from build123d import *
from OCP.BRepFilletAPI import BRepFilletAPI_MakeChamfer
from build123d.topology import SkipClean

# Parameters (mm, degrees)
SKETCH1_R                = 1.6
SKETCH1_W                = 16
SKETCH1_H                = 16
BOSS_EXTRUDE1_DEPTH      = 8
SKETCH2_W                = 16
SKETCH2_H                = 4
CUT_EXTRUDE1_DEPTH       = 40
FILLET1_R                = 4
BOSS_EXTRUDE5_DEPTH      = 12
BOSS_EXTRUDE5_DEPTH_BACK = 1
SKETCH3_W                = 32
SKETCH3_H                = 5
CHAMFER1_SIZE            = 3
CHAMFER2_SIZE            = 8
CHAMFER2_SIZE2           = 10
SKETCH5_W                = 12
SKETCH5_H                = 5
BOSS_EXTRUDE7_DEPTH      = 8
FILLET2_R                = 4
SKETCH6_R                = 1.6
CUT_EXTRUDE2_DEPTH       = 20
SKETCH7_R                = 3.05
CUT_EXTRUDE3_DEPTH       = 9
SKETCH8_R                = 3.05
BOSS_EXTRUDE8_DEPTH      = 5
BOSS_EXTRUDE9_START      = -5
SKETCH9_R                = 1.6
BOSS_EXTRUDE9_DEPTH      = 5
SKETCH10_R               = 5.55
CUT_EXTRUDE4_DEPTH       = 9
BOSS_EXTRUDE11_START     = 6
SKETCH11_R               = 5.55
BOSS_EXTRUDE11_DEPTH     = 6
SKETCH12_R               = 7.71946315
SKETCH12_R_2             = 3.05
BOSS_EXTRUDE12_DEPTH     = 5.5
SKETCH14_R               = 7
CUT_EXTRUDE6_DEPTH       = 1.5
CUT_EXTRUDE8_DEPTH       = 5
BOSS_EXTRUDE13_START     = -6
SKETCH19_R               = 2.06
SKETCH19_R_2             = 7
BOSS_EXTRUDE13_DEPTH     = 6
CUT_EXTRUDE9_DEPTH       = 8
FILLET3_R                = 2
CHAMFER3_SIZE            = 4


# Some blends are built 0.0001 mm under size
with BuildPart() as part:
    # Sketch1 → Boss-Extrude1 (new body)
    with BuildSketch(Plane(origin=(0, 0, 0), x_dir=(1, 0, 0), z_dir=(0, 1, 0))):
        with BuildLine():
            Line((-12, 16), (12, 16))
            ThreePointArc((12, 16), (14.828427125, 14.828427125), (16, 12))
            Line((16, 12), (16, -12))
            ThreePointArc((16, -12), (14.828427125, -14.828427125), (12, -16))
            Line((12, -16), (-12, -16))
            ThreePointArc((-12, -16), (-14.828427125, -14.828427125), (-16, -12))
            Line((-16, -12), (-16, 12))
            ThreePointArc((-16, 12), (-14.828427125, 14.828427125), (-12, 16))
        make_face()
        with Locations(Location((12, 12, 0), (0, 0, 270))):
            Circle(SKETCH1_R, mode=Mode.SUBTRACT)
        with Locations(Location((-12, 12, 0), (0, 0, 90))):
            Circle(SKETCH1_R, mode=Mode.SUBTRACT)
        with Locations(Location((12, -12, 0), (0, 0, 90))):
            Circle(SKETCH1_R, mode=Mode.SUBTRACT)
        with Locations(Location((-12, -12, 0), (0, 0, 270))):
            Circle(SKETCH1_R, mode=Mode.SUBTRACT)
        Rectangle(SKETCH1_W, SKETCH1_H, mode=Mode.SUBTRACT)
    extrude(amount=BOSS_EXTRUDE1_DEPTH)

    # Sketch2 → Cut-Extrude1 (cut)
    with BuildSketch(Plane(origin=(16, 0, 0), x_dir=(0, 0, -1), z_dir=(1, 0, 0))):
        with Locations((0, 2)):
            Rectangle(SKETCH2_W, SKETCH2_H)
    extrude(amount=-CUT_EXTRUDE1_DEPTH, mode=Mode.SUBTRACT)

    # Fillet1
    fillet1_edges = [part.edges().sort_by_distance(p)[0] for p in [
        (-16, 2, -8),
        (16, 2, -8),
        (-16, 2, 8),
        (16, 2, 8),
    ]]
    fillet(fillet1_edges, radius=FILLET1_R - 0.0001)  # a hair under: the kernel refuses the full size

    # Sketch3 → Boss-Extrude5 (add, two sides: drawn at the far end of the back side and taken through both)
    with BuildSketch(Plane(origin=(0, 8, 0), x_dir=(1, 0, 0), z_dir=(0, 1, 0)).offset(-BOSS_EXTRUDE5_DEPTH_BACK)):
        with Locations((0, 5.5)):
            Rectangle(SKETCH3_W, SKETCH3_H)
        with Locations((0, -5.5)):
            Rectangle(SKETCH3_W, SKETCH3_H)
    extrude(amount=BOSS_EXTRUDE5_DEPTH + BOSS_EXTRUDE5_DEPTH_BACK)

    # Chamfer1
    chamfer1_edges = [part.edges().sort_by_distance(p)[0] for p in [
        (8, 7, 5.5),
        (8, 7, -5.5),
        (-8, 7, -5.5),
        (-8, 7, 5.5),
    ]]
    chamfer(chamfer1_edges, length=CHAMFER1_SIZE - 0.0001)  # a hair under: the kernel refuses the full size

    # Chamfer2: one chamfer whose edges measure the first distance from different faces: ONE call of the kernel's chamfer builder (chamfer() names one face for all edges)
    chamfer2_edges_1 = [part.edges().sort_by_distance(p)[0] for p in [
        (-16, 20, -5.5),
        (-16, 20, 5.5),
    ]]
    chamfer2_side_1 = [part.faces().sort_by_distance(p)[0] for p in [
        (-16, 0.312409987, 11.99995),
    ]]
    chamfer2_edges_2 = [part.edges().sort_by_distance(p)[0] for p in [
        (16, 20, -5.5),
        (16, 20, 5.5),
    ]]
    chamfer2_side_2 = [part.faces().sort_by_distance(p)[0] for p in [
        (16, 0.312409987, -11.99995),
    ]]
    chamfer2 = BRepFilletAPI_MakeChamfer(part.part.solid().wrapped)
    for e in chamfer2_edges_1:
        chamfer2.Add(CHAMFER2_SIZE, CHAMFER2_SIZE2, e.wrapped, chamfer2_side_1[0].wrapped)  # the first distance lies on this face
    for e in chamfer2_edges_2:
        chamfer2.Add(CHAMFER2_SIZE, CHAMFER2_SIZE2, e.wrapped, chamfer2_side_2[0].wrapped)  # the first distance lies on this face
    add(Compound.cast(chamfer2.Shape()), mode=Mode.REPLACE)

    # Sketch5 → Boss-Extrude7 (add)
    with BuildSketch(Plane(origin=(0, 20, 0), x_dir=(1, 0, 0), z_dir=(0, 1, 0))):
        with Locations((0, 5.5)):
            Rectangle(SKETCH5_W, SKETCH5_H)
        with Locations((0, -5.5)):
            Rectangle(SKETCH5_W, SKETCH5_H)
    extrude(amount=BOSS_EXTRUDE7_DEPTH)

    # Fillet2
    fillet2_edges = [part.edges().sort_by_distance(p)[0] for p in [
        (-6, 28, -5.5),
        (6, 28, -5.5),
        (-6, 28, 5.5),
        (6, 28, 5.5),
    ]]
    fillet(fillet2_edges, radius=FILLET2_R)

    # Sketch6 → Cut-Extrude2 (cut)
    with BuildSketch(Plane.XY.offset(8)):
        with Locations((0, 24)):
            Circle(SKETCH6_R)
    extrude(amount=-CUT_EXTRUDE2_DEPTH, mode=Mode.SUBTRACT)

    # Sketch7 → Cut-Extrude3 (cut)
    with BuildSketch(Plane.XY.offset(8)):
        with Locations((0, 24)):
            Circle(SKETCH7_R)
    extrude(amount=-CUT_EXTRUDE3_DEPTH, mode=Mode.SUBTRACT)

    # Sketch8 → Boss-Extrude8 (add)
    with BuildSketch(Plane.XY.offset(8)):
        with BuildLine():
            Line((-9, 24), (-9, 15))
            Line((-9, 15), (0, 15))
            Line((0, 15), (9, 15))
            Line((9, 15), (9, 24))
            ThreePointArc((9, 24), (0, 33), (-9, 24))
        make_face()
        with Locations((0, 24)):
            Circle(SKETCH8_R, mode=Mode.SUBTRACT)
    extrude(amount=-BOSS_EXTRUDE8_DEPTH)

    # Sketch9 → Boss-Extrude9 (add)
    with BuildSketch(Plane(origin=(0, 0, -8), x_dir=(-1, 0, 0), z_dir=(0, 0, -1)).offset(BOSS_EXTRUDE9_START)):
        with BuildLine():
            Line((-9, 24), (-9, 11))
            Line((-9, 11), (9, 11))
            Line((9, 11), (9, 24))
            ThreePointArc((9, 24), (0, 33), (-9, 24))
        make_face()
        with Locations(Location((0, 24, 0), (0, 0, 180))):
            Circle(SKETCH9_R, mode=Mode.SUBTRACT)
    extrude(amount=BOSS_EXTRUDE9_DEPTH)

    # Sketch10 → Cut-Extrude4 (cut)
    with BuildSketch(Plane(origin=(0, 0, -8), x_dir=(-1, 0, 0), z_dir=(0, 0, -1))):
        with Locations((0, 24)):
            Circle(SKETCH10_R)
    extrude(amount=-CUT_EXTRUDE4_DEPTH, mode=Mode.SUBTRACT)

    # Sketch11 → Boss-Extrude11 (add)
    with SkipClean():  # the faces are left unmerged after this step: merging them gives an invalid solid
        with BuildSketch(Plane.XY.offset(-3).offset(BOSS_EXTRUDE11_START)):
            with BuildLine():
                Line((-9, 24), (-9, 17.6))
                Line((-9, 17.6), (-16, 12))
                Line((-16, 12), (-16, 8))
                Line((-16, 8), (-8, 8))
                Line((-8, 8), (-8, 4))
                Line((-8, 4), (-5, 7))
                Line((-5, 7), (5, 7))
                Line((5, 7), (8, 4))
                Line((8, 4), (8, 8))
                Line((8, 8), (16, 8))
                Line((16, 8), (16, 12))
                Line((16, 12), (9, 17.6))
                Line((9, 17.6), (9, 24))
                ThreePointArc((9, 24), (0, 33), (-9, 24))
            make_face()
            with Locations(Location((0, 24, 0), (0, 0, 180))):
                Circle(SKETCH11_R, mode=Mode.SUBTRACT)
        extrude(amount=-BOSS_EXTRUDE11_DEPTH)

    # Sketch12 → Boss-Extrude12 (add)
    with BuildSketch(Plane(origin=(0, 0, 3), x_dir=(-1, 0, 0), z_dir=(0, 0, -1))):
        with Locations((0, 24)):
            Circle(SKETCH12_R)
        with Locations(Location((0, 24, 0), (0, 0, 180))):
            Circle(SKETCH12_R_2, mode=Mode.SUBTRACT)
    extrude(amount=BOSS_EXTRUDE12_DEPTH)

    # Sketch14 → Cut-Extrude6 (cut)
    with BuildSketch(Plane(origin=(0, 0, -8), x_dir=(-1, 0, 0), z_dir=(0, 0, -1))):
        with Locations((0, 24)):
            Circle(SKETCH14_R)
    extrude(amount=-CUT_EXTRUDE6_DEPTH, mode=Mode.SUBTRACT)

    # Sketch16 → Cut-Extrude8 (cut)
    with SkipClean():  # the faces are left unmerged after this step: merging them gives an invalid solid
        with BuildSketch(Plane.XY.offset(8)):
            Polygon((-16, 8), (16, 8), (29.507054263, 32.870046285), (-4.901166162, 51.167615183), (-28.978076235, 29.234025221), align=None)
        extrude(amount=-CUT_EXTRUDE8_DEPTH, mode=Mode.SUBTRACT)

    # Sketch19 → Boss-Extrude13 (add)
    with SkipClean():  # the faces are left unmerged after this step: merging them gives an invalid solid
        with BuildSketch(Plane(origin=(0, 0, -8), x_dir=(-1, 0, 0), z_dir=(0, 0, -1)).offset(BOSS_EXTRUDE13_START)):
            with BuildLine():
                Line((16.13, 29), (7.483314774, 29))
                ThreePointArc((7.483314774, 29), (0, 33), (-7.483314774, 29))
                Line((-7.483314774, 29), (-16.13, 29))
                ThreePointArc((-16.13, 29), (-20.352655353, 26.677532777), (-20.652519245, 21.867672708))
                Line((-20.652519245, 21.867672708), (-16, 12))
                Line((-16, 12), (16, 12))
                Line((16, 12), (20.652519245, 21.867672708))
                ThreePointArc((20.652519245, 21.867672708), (20.352655353, 26.677532777), (16.13, 29))
            make_face()
            with Locations((16.13, 24)):
                Circle(SKETCH19_R, mode=Mode.SUBTRACT)
            with Locations(Location((-16.13, 24, 0), (0, 0, 180))):
                Circle(SKETCH19_R, mode=Mode.SUBTRACT)
            with Locations((0, 24)):
                Circle(SKETCH19_R_2, mode=Mode.SUBTRACT)
        extrude(amount=BOSS_EXTRUDE13_DEPTH)

    # Sketch21 → Cut-Extrude9 (cut)
    with SkipClean():  # the faces are left unmerged after this step: merging them gives an invalid solid
        with BuildSketch(Plane(origin=(0, 0, -16), x_dir=(-1, 0, 0), z_dir=(0, 0, -1))):
            with BuildLine():
                Line((8, 8), (0, 8))
                Line((0, 8), (0, 3))
                ThreePointArc((0, 3), (4.716990566, 4.352815094), (8, 8))
            make_face()
            with BuildLine():
                Line((0, 3), (0, 8))
                Line((0, 8), (-8, 8))
                ThreePointArc((-8, 8), (-4.716990566, 4.352815094), (0, 3))
            make_face()
        extrude(amount=-CUT_EXTRUDE9_DEPTH, mode=Mode.SUBTRACT)

    # Fillet3
    # the kernel refuses this fillet: 2 mm, written as the material it takes off along each edge
    with BuildSketch(Plane(origin=(8, 8, -18.912878475), x_dir=(1, 0, 0), z_dir=(0, 0, 1))) as fillet3_piece_1:
        with BuildLine():
            CenterArc((1.16515139, -2), FILLET3_R, 90, 57.22888336)
            ThreePointArc((-0.516527764, -0.917431193), (-0.244685814, -0.466360256), (0, 0))
            Line((0, 0), (1.16515139, 0))
        make_face()
    extrude(amount=10.912878475, mode=Mode.SUBTRACT)
    with BuildSketch(Plane(origin=(-8, 8, -18.912878475), x_dir=(-1, 0, 0), z_dir=(0, 0, 1))) as fillet3_piece_2:
        with BuildLine():
            CenterArc((1.16515139, 2), FILLET3_R, 212.77111664, 57.22888336)
            ThreePointArc((-0.516527764, 0.917431193), (-0.244685814, 0.466360256), (0, 0))
            Line((0, 0), (1.16515139, 0))
        make_face()
    extrude(amount=10.912878475, mode=Mode.SUBTRACT)

    # Chamfer3
    chamfer3_edges = [part.edges().sort_by_distance(p)[0] for p in [
        (0, 8, 3),
    ]]
    chamfer(chamfer3_edges, length=CHAMFER3_SIZE)


solid = part.part
Geometry: final body of the model. Coordinates: model frame, mm. A direction names the side the tool comes from. Give positions to 0.01 mm unless a question says otherwise; leave off trailing zeros. Loops run counter-clockwise (first coordinate to the right, second up) from the corner with the lowest first, then second, coordinate; pieces in that order, holes last. Notation, with made-up numbers: (30.25, 43) - (64.25, 43) arc R18 cw to (64.25, 77) - close; hole circle Ø4 at (66.25, 82.25). An arc over 180 degrees is marked (long way). One line per question, with ' | ' between items. Start each with the question number.
(1) Section query A-A on z = 2.5. Return loops of the section in (x, y).
(2) Ray query, line 1 (X direction, y = 5, z = 12); line 2 (Z direction, x = -7.5, y = 3); line 3 (Y direction, x = 0, z = -7.05). Return the intervals inside material, ascending. Write a range as from..to.
(3) Section query D-D on x = 4.5. Return loops of the section in (y, z), then the cut area to 3 significant figures.
(4) Section query B-B on x = -17. Return loops of the section in (y, z), then the cut area to 3 significant figures.
(5) Section query C-C on z = 11.5. Count the separate pieces of the cut face and the enclosed holes in it, then the cut area to 3 significant figures.
(6) Contact query for flat-ended pins moving along their axis: pin 1 (6 mm diameter, centred on y = 8, z = 1, fed in from -X); pin 2 (10 mm diameter, centred on x = -8, z = 2.5, fed in from +Y); pin 3 (11 mm diameter, centred on x = 0, y = 24, fed in from +Z). Output: stop coordinate, or through.
(7) Pull-direction query (X, two-part tool) for faces 1 (the flat face through (-9, 21, 1)), 2 (the flat face through (0, 0, -12)), 3 (the cylindrical face through (-17.08, 22.17, -4.96)); classes: released by +X, released by -X, zero draft, split by the parting line, or undercut.
(8) Reachability of faces 4 (the flat face through (14, 23, -2)), 5 (the flat face through (16, 7, 0)), 6 (the cylindrical face through (14.797, 2.028, 9.141)), 7 (the flat face through (0, 7, 0)), 8 (the cylindrical face through (0.722, 18.497, -4.472)) from +Z, -Z, +X, -X, +Y, -Y: full face, straight path, thin tool, end or side. Return the list, or none.
The answers:
1) outline: (-16, 4) - (-8, 4) - (-5, 7) - (5, 7) - (8, 4) - (16, 4) - (16, 12) - (9, 17.6) - (9, 24) arc R9 ccw to (-9, 24) - (-9, 17.6) - (-16, 12) - close; hole circle Ø6.1 at (0, 24)
2) line 1: -16..-13.6, -10.4..10.4, 13.6..16 | line 2: -16..-8, 8..16 | line 3: 7..17, 31..33
3) outline: (0, -16) - (4.22, -16) - (4.22, -8) - (0, -8) - close; (0, 8) - (7, 8) - (7, -8) - (18.64, -8) - (18.64, -6.5) - (20.75, -6.5) - (20.75, -2.5) - (27.25, -2.5) - (27.25, -6.5) - (29.36, -6.5) - (29.36, -8) - (31.79, -8) - (31.79, 3) - (12, 3) - (8, 7) - (8, 16) - (0, 16) - close | area: 341 mm2
4) outline: (14.12, -8) - (22.13, -8) - (22.13, -2) - (14.12, -2) - close; (25.87, -8) - (28.92, -8) - (28.92, -2) - (25.87, -2) - close | area: 66.4 mm2
5) separate pieces: 3 | enclosed holes: 0 | area: 207 mm2
6) pin 1: x = -16 | pin 2: y = 32.49 | pin 3: z = 3
7) face 1: released by -X | face 2: zero draft | face 3: undercut
8) face 4: +Z, +X, +Y | face 5: +Z, -Z, +X, -Y | face 6: +X, -Y | face 7: -Z, -Y | face 8: -Z
